Check sheet for the modelled part. Datum: model origin and axes. Units: mm. Face numbers are marked on the shaded views. A direction names the side the tool comes from. Round coordinates to 2 decimals unless told otherwise and drop trailing zeros. Write each loop counter-clockwise with the first axis right and the second up, starting at its lowest first coordinate (ties: lowest second). Pieces come first, ordered by that corner, then holes. Notation, with made-up numbers: (44.5, 1.25) -> (49.5, 1.25) arc R20 cw to (49.5, 33.25) -> close; hole circle Ø9 at (-36.75, 59). An arc over 180 degrees is marked (long way). One line per item, written item: value.
Autodesk Fusion 360 part; units mm, degrees
sketch "Sketch1" plane through (0, 0, 0) normal (0, 1, 0) x (1, 0, 0)
  line L0 (0, 0) -> (22, 0)
  line L1 (22, 0) -> (22, 28)
  line L2 (22, 28) -> (0, 28)
  line L3 (0, 28) -> (0, 0)
  line L4 (11, 0) -> (11, 0.5)
  line L5 (11, 0.5) -> (2, 0.5)
  circle A0 centre (2, 1.8) radius 1.3
  line L6 (2, 1.8) -> (2, 12.8)
  circle A1 centre (2, 12.8) radius 1.3
  circle A2 centre (20, 1.8) radius 1.3
  circle A3 centre (20, 12.8) radius 1.3
  line L7 (2, 7.3) -> (22, 7.3)
  line L8 (2, 7.3) -> (0, 7.3)
  line L9 (0, 7.3) -> (0, 5.3)
  line L10 (0, 5.3) -> (22, 5.3)
  line L11 (0, 7.3) -> (0, 9.3)
  line L12 (0, 9.3) -> (22, 9.3)
  dimension "d1" = 22
  dimension "d2" = 28
  dimension "d3" = 0.5
  dimension "d4" = 9
  dimension "d5" = 2.6
  dimension "d6" = 11
  dimension "d7" = 2.6
  dimension "d8" = 2
  dimension "d9" = 2
extrude "Extrude1" add sketch "Sketch1" against normal blind 1.5 contours L0 L3 L4 L5 A0 L6 L10 | L0 L1 L4 L5 A0 L6 L10 | L3 L6 L8 L9 L10 | L3 L6 L8 L11 L12 | L1 L6 L7 L10 | L1 L2 L3 L12 | L1 L6 L7 L12
extrude "Extrude2" add sketch "Sketch1" along normal blind 1 contours L3 L6 L8 L9 L10 | L3 L6 L8 L11 L12 | L1 L6 L7 L10 | L1 L6 L7 L12
chamfer "Chamfer1" distance 0.5 angle 45 2 edges at (11, 1, -5.3) (11, 1, -9.3)
equation "d4 = ( 18 / 2 ) * 1 mm"
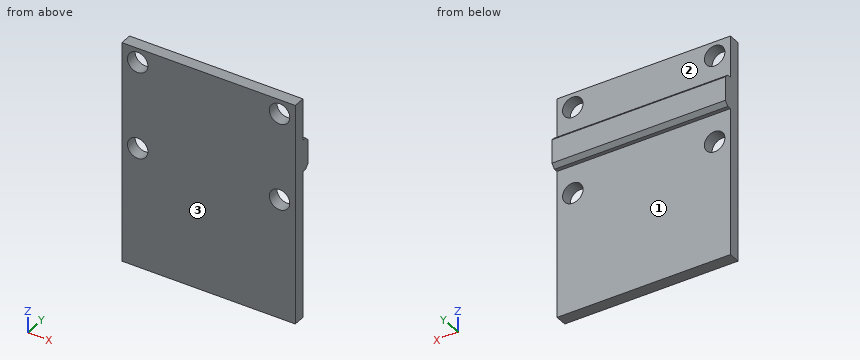
Item 1: Sectioned sample at A-A on x = 20. Enter the section's corners in (y, z).
Answer:
outline: (-1.5, -28) -> (0, -28) -> (0, -14.1) -> (-1.5, -14.1) -> close; (-1.5, -11.5) -> (0, -11.5) -> (0, -9.3) -> (0.5, -9.3) -> (1, -8.8) -> (1, -5.8) -> (0.5, -5.3) -> (0, -5.3) -> (0, -3.1) -> (-1.5, -3.1) -> close; (-1.5, -0.5) -> (0, -0.5) -> (0, 0) -> (-1.5, 0) -> close
Item 2: Sectioned sample at B-B on z = -12.8. Enter the section's corners in (x, y).
Answer:
outline: (0, -1.5) -> (0.7, -1.5) -> (0.7, 0) -> (0, 0) -> close; (3.3, -1.5) -> (18.7, -1.5) -> (18.7, 0) -> (3.3, 0) -> close; (21.3, -1.5) -> (22, -1.5) -> (22, 0) -> (21.3, 0) -> close
Item 3: Depth check by flat-ended pin: P1, Ø10, axis at x = 6.5, z = -16, coming from the +Y side. Enter the tip coordinate at first touch or a pass-through.
Answer:
P1: stops at y = 0
Item 4: Thickness scan on line 1 (X direction, y = -1, z = -12.8); line 2 (Z direction, x = 2, y = -0.95); line 3 (Z direction, x = 2.5, y = -0.3). Record the ranges inside material, lowest first.
Answer:
line 1: x = 0 to 0.7, 3.3 to 18.7, 21.3 to 22
line 2: z = -28 to -14.1, -11.5 to -3.1, -0.5 to 0
line 3: z = -28 to -14, -11.6 to -3, -0.6 to 0
Item 5: Sectioned sample at D-D on x = 16.5. Enter the section's corners in (y, z).
Answer:
outline: (-1.5, -28) -> (0, -28) -> (0, -9.3) -> (0.5, -9.3) -> (1, -8.8) -> (1, -5.8) -> (0.5, -5.3) -> (0, -5.3) -> (0, 0) -> (-1.5, 0) -> close
Item 6: Sectioned sample at C-C on y = -0.6. Enter the section's corners in (x, z), and give its area (3 significant figures).
Answer:
outline: (0, -28) -> (22, -28) -> (22, 0) -> (0, 0) -> close; hole circle Ø2.6 at (2, -12.8); hole circle Ø2.6 at (2, -1.8); hole circle Ø2.6 at (20, -12.8); hole circle Ø2.6 at (20, -1.8)
area: 595 mm^2
Item 7: Tool access check on the marked faces 1, 2 and 3. Record the directions out of +Z, -Z, +X, -X, +Y, -Y that give a thin tool (end or side, any length) a straight path to the whole face; none if there is none.
Answer:
face 1: -Z, +X, -X, +Y
face 2: +Z, +X, -X, +Y
face 3: +Z, -Z, +X, -X, -Y
